Source: three-view drawing plus pictorial views. Frame: mm from the lowest corner of the part. Give positions to 0.01 mm unless a question says otherwise; leave off trailing zeros. Order: outer loops, then holes, each group sorted by start corner. A loop starts at its lowest first (then second) coordinate and runs counter-clockwise, first axis right, second up. Notation, with made-up numbers: (81, 41) - (128, 41) arc R26 cw to (128, 64) - close; hole circle Ø6 at (-4.5, 58.25). An arc over 180 degrees is marked (long way). Use CSV: the item, a comma, the result in double quotes.
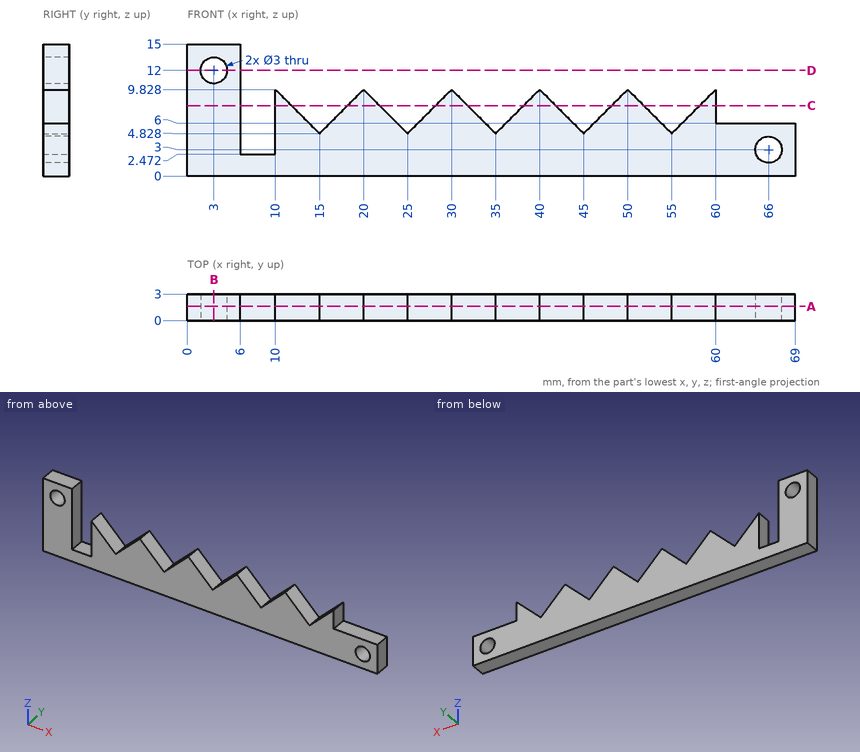
Item 1: Section B-B on x = 3. Return the cut outline in (y, z), then the cut area to 3 significant figures.
Filled in:
outline,"(0, 0) - (3, 0) - (3, 10.5) - (0, 10.5) - close; (0, 13.5) - (3, 13.5) - (3, 15) - (0, 15) - close"
area,"36.0 mm2"
Item 2: Section A-A on y = 1.6. Return the cut outline in (x, z), then the cut area to 3 significant figures.
Filled in:
outline,"(0, 0) - (69, 0) - (69, 6) - (60, 6) - (60, 9.83) - (55, 4.83) - (50, 9.83) - (45, 4.83) - (40, 9.83) - (35, 4.83) - (30, 9.83) - (25, 4.83) - (20, 9.83) - (15, 4.83) - (10, 9.83) - (10, 2.47) - (6, 2.47) - (6, 15) - (0, 15) - close; hole circle Ø3 at (3, 12); hole circle Ø3 at (66, 3)"
area,"506 mm2"
Item 3: Section C-C on z = 8. Return the cut outline in (x, y).
Filled in:
outline,"(0, 0) - (6, 0) - (6, 3) - (0, 3) - close; (10, 0) - (11.83, 0) - (11.83, 3) - (10, 3) - close; (18.17, 0) - (21.83, 0) - (21.83, 3) - (18.17, 3) - close; (28.17, 0) - (31.83, 0) - (31.83, 3) - (28.17, 3) - close; (38.17, 0) - (41.83, 0) - (41.83, 3) - (38.17, 3) - close; (48.17, 0) - (51.83, 0) - (51.83, 3) - (48.17, 3) - close; (58.17, 0) - (60, 0) - (60, 3) - (58.17, 3) - close"
Item 4: Material intervals for line 1 (X direction, y = 0.55, z = 3); line 2 (Z direction, x = 3, y = 2.3); line 3 (X direction, y = 2, z = 12), sorted ascending. Write a range as from..to.
Filled in:
line 1,"x = 0..6, 10..64.5, 67.5..69"
line 2,"z = 0..10.5, 13.5..15"
line 3,"x = 0..1.5, 4.5..6"
Item 5: First-contact query: pin 1 (1.5 mm diameter, centred on x = 8, y = 1, fed in from +Z); pin 2 (0.9 mm diameter, centred on y = 1, z = 9.5, fed in from +X); pin 3 (1.5 mm diameter, centred on x = 63, y = 1, fed in from +Z). Flat tips, straight axial feed; report the tip coordinate or a pass-through.
Filled in:
pin 1,"stops at z = 2.47"
pin 2,"stops at x = 60"
pin 3,"stops at z = 6"
Item 6: Section D-D on z = 12. Return the cut outline in (x, y).
Filled in:
outline,"(0, 0) - (1.5, 0) - (1.5, 3) - (0, 3) - close; (4.5, 0) - (6, 0) - (6, 3) - (4.5, 3) - close"
